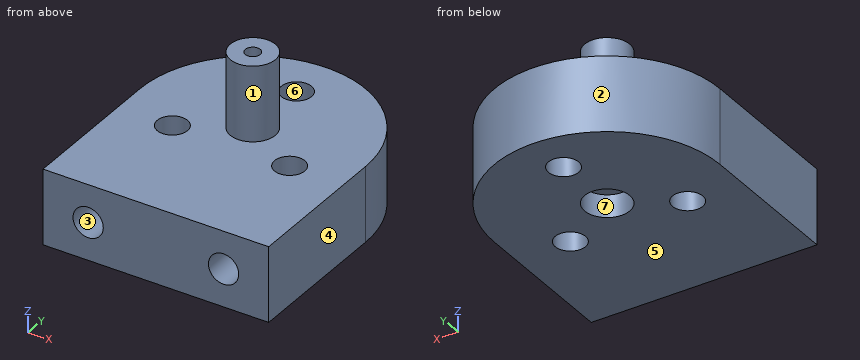
Autodesk Inventor part; units mm, degrees
ref_plane "Work Plane1" through (-7.5, 10, 10) normal (1, 0, 0) x (0, 0, -1)
ref_plane "YZ Plane" through (0, 0, 0) normal (1, 0, 0) x (0, 1, 0)
ref_plane "XZ Plane" through (0, 0, 0) normal (0, 1, 0) x (-1, 0, 0)
sketch "Sketch1" plane through (0, 0, 0) normal (0, 0, 1) x (1, 0, 0)
  line L0 (0, 0) -> (-15, 0)
  line L1 (-15, 0) -> (-15, 10)
  line L2 (-15, 10) -> (0, 10)
  line L3 (0, 10) -> (0, 0)
  circle A0 centre (-7.5, 10) radius 7.5
  dimension "d0" = 15
  dimension "d1" = 10
extrude "Extrusion1" add sketch "Sketch1" along normal blind 5
sketch "Sketch2" plane through (0, 0, 5) normal (0, 0, 1) x (1, 0, 0)
  arc A0 (0, 10) -> (-15, 10) centre (-7.5, 10) ccw
  circle A1 centre (-7.5, 10) radius 1.5
  point P0 (0, 0)
  dimension "d4" = 3
extrude "Extrusion2" add sketch "Sketch2" along normal blind 5
sketch "Sketch3" plane through (-7.5, 10, 10) normal (0, 0, 1) x (1, 0, 0)
  point P0 (7.5, -10)
  point P1 (0, 0)
  point P2 (0, 0)
hole "Hole1" at (-7.5, 10, 10) direction (0, 0, -1) diameter 1 end through all
sketch "Sketch4" plane through (0, 0, 0) normal (0, 0, -1) x (-1, 0, 0)
  circle A0 centre (7.5, 10) radius 0.5
  circle A1 centre (7.5, 10) radius 0.9
  point P0 (0, 0)
  dimension "d14" = 1.8
extrude "Extrusion3" cut sketch "Sketch4" against normal blind 7 contours A0 | A1
sketch "Sketch5" plane through (0, 0, 0) normal (0, 0, -1) x (-1, 0, 0)
  circle A0 centre (7.5, 10) radius 0.9
  circle A1 centre (7.5, 10) radius 1.5
  point P0 (0, 0)
  dimension "d17" = 3
extrude "Extrusion4" cut sketch "Sketch5" against normal blind 1.5
sketch "Sketch7" plane through (-15, 0, 0) normal (0, -1, 0) x (1, 0, 0)
  line L0 (15, 0) -> (15, 5)
  line L1 (0, 0) -> (0, 5)
  line L2 (0, 0) -> (15, 0)
  point P0 (12, 2.5)
  point P1 (3, 2.5)
  dimension "d21" = 3
  dimension "d22" = 3
  dimension "d23" = 2.5
  dimension "d24" = 2.5
hole "Hole2" at (-3, 0, 2.5) at (-12, 0, 2.5) direction (0, 1, 0) diameter 2.013 depth 4 tip angle 118
sketch "Sketch8" plane through (0, 0, 0) normal (0, 0, -1) x (-1, 0, 0)
  circle A0 centre (7.5, 10) radius 0.5
  circle A1 centre (7.5, 10) radius 4.5 construction
  point P0 (0, 0)
  point P1 (7.5, 14.5)
  point P2 (11.3971, 7.75)
  point P3 (3.6029, 7.75)
  dimension "d32" = 9
  dimension "d33" = 120
  dimension "d34" = 120
hole "Hole3" at (-7.5, 14.5, 0) at (-11.3971, 7.75, 0) at (-3.6029, 7.75, 0) direction (0, 0, 1) diameter 2.013 end through all
sketch "Sketch9" plane through (-7.5, 10, 10) normal (0, 0, 1) x (1, 0, 0)
  circle A0 centre (0, 0) radius 0.9
  point P0 (7.5, -10)
ref_plane "Work Plane1" through (-7.5, 10, 10) normal (1, 0, 0) x (0, 0, -1)
properties part number "FillLine-SealFlange" material "Brass, Soft Yellow"
The listing builds one solid part. Answer for the finished solid, in the listing's coordinates (mm). Face numbers are marked on the shaded views. A direction names the side the tool comes from. Round coordinates to 2 decimals unless told otherwise and drop trailing zeros. Order: outer loops, then holes, each group sorted by start corner. A loop starts at its lowest first (then second) coordinate and runs counter-clockwise, first axis right, second up. Notation, with made-up numbers: (-3, 59) -> (45, 59) arc R21 cw to (45, 70) -> close; hole circle Ø11 at (78.5, 78.5). An arc over 180 degrees is marked (long way). Write each question's results on one line, items separated by ' | '. Start each with the question number.
Q1. Find section B-B (y = 2). Determine the outline of the cut face in (x, z).
Q2. Find section A-A (y = 7.75). Determine the outline of the cut face in (x, z).
Q3. Find section D-D (z = 4.5). Determine the outline of the cut face in (x, y).
Q4. Each of these flat-tipped pins is pushed along its axis until it touches: pin 1 (5 mm diameter, centred on x = -6.5, z = 9, fed in from -Y); pin 2 (3 mm diameter, centred on x = -12.5, y = 5.5, fed in from +Z); pin 3 (1 mm diameter, centred on x = -9, z = 7.5, fed in from +Y). Where does it stop, or does it pass through?
Q5. Which of the six approach directions +Z, -Z, +X, -X, +Y, -Y give full straight-line access (tool end or side, diameter ignored) to the marked faces 1, 2 and 3?
Q6. Find section C-C (z = 7.75). Determine the outline of the cut face in (x, y), then the cut area to 3 significant figures.
Q7. Straight lines are drawn through the part: probe 1 along Y at (x, z) = (-7.5, 4); probe 2 along X at (y, z) = (7.75, 3.5); probe 3 along X at (y, z) = (2.35, 2.5). For each, find the intervals that lie inside material, in ascending order. Write a range as from..to.
Q8. The mould has two halves that part along X. Classify the marked faces 4, 5, 6 and 7: pulls with the +X half, pulls with the -X half, needs draft (parallel to the pull), parting line crosses it, or undercut.
Worked answers:
1) outline: (-15, 0) -> (0, 0) -> (0, 5) -> (-15, 5) -> close; hole circle Ø2.01 at (-12, 2.5); hole circle Ø2.01 at (-3, 2.5)
2) outline: (-15, 0) -> (-12.4, 0) -> (-12.4, 5) -> (-15, 5) -> close; (-10.39, 0) -> (-4.61, 0) -> (-4.61, 5) -> (-10.39, 5) -> close; (-2.6, 0) -> (0, 0) -> (0, 5) -> (-2.6, 5) -> close
3) outline: (-15, 0) -> (0, 0) -> (0, 10) arc R7.5 ccw to (-15, 10) -> close; hole circle Ø2.01 at (-11.4, 7.75); hole circle Ø2.01 at (-7.5, 14.5); hole circle Ø1.8 at (-7.5, 10); hole circle Ø2.01 at (-3.6, 7.75)
4) pin 1: stops at y = 8.5 | pin 2: stops at z = 5 | pin 3: stops at y = 11.12
5) face 1: +Z | face 2: +Z, -Z, +Y | face 3: -Y
6) outline: circle Ø3 at (-7.5, 10); hole circle Ø1 at (-7.5, 10) | area: 6.28 mm2
7) probe 1: y = 0..9.1, 10.9..13.49, 15.51..17.5 | probe 2: x = -15..-12.4, -10.39..-4.61, -2.6..0 | probe 3: x = -15..-13.01, -10.99..-4.01, -1.99..0
8) face 4: pulls with the +X half | face 5: needs draft | face 6: undercut | face 7: undercut
